from build123d import *

# Parameters (mm, degrees)
F0_R     = 76.2
F1_DEPTH = 25.4
F3_DEPTH = 25.4


with BuildPart() as f1:
    # F0 (on Front) → F1 (new body)
    with BuildSketch(Plane.XZ):
        Circle(F0_R)
    extrude(amount=F1_DEPTH)

    # F2 (on face) → F3 (cut)
    with BuildSketch(Plane.XZ.offset(25.4)):
        with BuildLine():
            Line((-52.494522, 25.127975), (-38.677355, 18.514))
            ThreePointArc((-38.677355, 18.514), (-35.080153, 18.213926), (-32.19177, 20.37891))
            ThreePointArc((-32.19177, 20.37891), (-26.940768, 26.940768), (-20.37891, 32.19177))
            ThreePointArc((-20.37891, 32.19177), (-18.213926, 35.080153), (-18.514, 38.677355))
            Line((-18.514, 38.677355), (-25.127975, 52.494522))
            ThreePointArc((-25.127975, 52.494522), (-28.231073, 55.161107), (-32.293557, 54.675188))
            ThreePointArc((-32.293557, 54.675188), (-44.901281, 44.901281), (-54.675188, 32.293557))
            ThreePointArc((-54.675188, 32.293557), (-55.161107, 28.231073), (-52.494522, 25.127975))
        make_face()
        with BuildLine():
            Line((19.351072, -54.887394), (14.257645, -40.440395))
            ThreePointArc((14.257645, -40.440395), (11.926223, -37.684605), (8.352953, -37.173084))
            ThreePointArc((8.352953, -37.173084), (0, -38.1), (-8.352953, -37.173084))
            ThreePointArc((-8.352953, -37.173084), (-11.926223, -37.684605), (-14.257645, -40.440395))
            Line((-14.257645, -40.440395), (-19.351072, -54.887394))
            ThreePointArc((-19.351072, -54.887394), (-19.04241, -58.967176), (-15.826203, -61.496189))
            ThreePointArc((-15.826203, -61.496189), (0, -63.5), (15.826203, -61.496189))
            ThreePointArc((15.826203, -61.496189), (19.04241, -58.967176), (19.351072, -54.887394))
        make_face()
        with BuildLine():
            Line((25.127975, 52.494522), (18.514, 38.677355))
            ThreePointArc((18.514, 38.677355), (18.213926, 35.080153), (20.37891, 32.19177))
            ThreePointArc((20.37891, 32.19177), (26.940768, 26.940768), (32.19177, 20.37891))
            ThreePointArc((32.19177, 20.37891), (35.080153, 18.213926), (38.677355, 18.514))
            Line((38.677355, 18.514), (52.494522, 25.127975))
            ThreePointArc((52.494522, 25.127975), (55.161107, 28.231073), (54.675188, 32.293557))
            ThreePointArc((54.675188, 32.293557), (44.901281, 44.901281), (32.293557, 54.675188))
            ThreePointArc((32.293557, 54.675188), (28.231073, 55.161107), (25.127975, 52.494522))
        make_face()
    extrude(amount=-F3_DEPTH, mode=Mode.SUBTRACT)


solid = f1.part
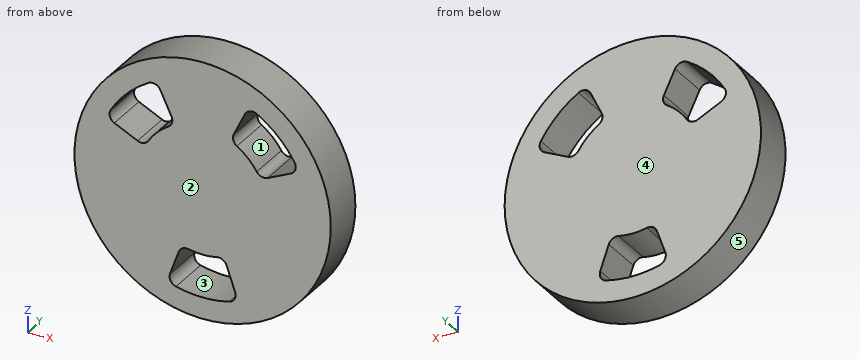
Could you check a few things on this model? Use its own coordinates, in mm. Face numbers are marked on the shaded views. A direction names the side the tool comes from. Give positions to 0.01 mm unless a question says otherwise; leave off trailing zeros. Order: outer loops, then holes, each group sorted by start corner. A loop starts at its lowest first (then second) coordinate and runs counter-clockwise, first axis right, second up.
1. I need wall thicknesses on L1, parallel to X at y = -20.25, z = 41; L2, parallel to X at y = -11.75, z = 30.5; L3, parallel to Z at x = 33, y = -1.75. Which ranges of each line are inside material? Lowest first, please.
Answers below:
L1: x = -64.23 to -48.49, -19.63 to 19.63, 48.49 to 64.23
L2: x = -69.83 to -55.32, -22.83 to 22.83, 55.32 to 69.83
L3: z = -68.68 to 19.4, 54.25 to 68.68
2. Suppose I cut it at A-A (x = 0). Write out the boundary of the cut face in (y, z), plus the area to 3 significant figures.
Answers below:
outline: (-25.4, -76.2) - (0, -76.2) - (0, -63.5) - (-25.4, -63.5) - close; (-25.4, -38.1) - (0, -38.1) - (0, 76.2) - (-25.4, 76.2) - close
area: 3,230 mm2
3. For pin 1 (1.5 mm diameter, centred on x = -28, y = -21.5, fed in from -Z); pin 2 (1.5 mm diameter, centred on y = -15, z = -47.5, fed in from -X); pin 3 (6 mm diameter, centred on x = 0, y = -12, fed in from +Z), each with a flat end and sliding along its axis, tell me the tip position at first contact or that it passes through.
Answers below:
pin 1: stops at z = -71.16
pin 2: stops at x = -60.17
pin 3: stops at z = 76.2
4. Thinking about a two-plate mould opening in Z: for the marked faces 3, 4 and 5, which applies, +Z half, -Z half, draft (parallel to the pull), parting line (faces both ways), or undercut?
Answers below:
face 3: undercut
face 4: draft
face 5: parting line
5. Suppose I cut it at C-C (x = -44.5). Write out the boundary of the cut face in (y, z).
Answers below:
outline: (-25.4, -61.86) - (0, -61.86) - (0, 21.3) - (-25.4, 21.3) - close; (-25.4, 45.3) - (0, 45.3) - (0, 61.86) - (-25.4, 61.86) - close
6. Suppose I cut it at B-B (y = -5.5). Write out the boundary of the cut face in (x, z), plus the area to 3 significant figures.
Answers below:
outline: circle Ø152.4 at (0, 0); hole (-54.68, 32.29) arc R5.08 ccw to (-52.49, 25.13) - (-38.68, 18.51) arc R5.08 ccw to (-32.19, 20.38) arc R38.1 cw to (-20.38, 32.19) arc R5.08 ccw to (-18.51, 38.68) - (-25.13, 52.49) arc R5.08 ccw to (-32.29, 54.68) arc R63.5 ccw to start; hole (-19.35, -54.89) arc R5.08 ccw to (-15.83, -61.5) arc R63.5 ccw to (15.83, -61.5) arc R5.08 ccw to (19.35, -54.89) - (14.26, -40.44) arc R5.08 ccw to (8.35, -37.17) arc R38.1 cw to (-8.35, -37.17) arc R5.08 ccw to (-14.26, -40.44) - close; hole (18.51, 38.68) arc R5.08 ccw to (20.38, 32.19) arc R38.1 cw to (32.19, 20.38) arc R5.08 ccw to (38.68, 18.51) - (52.49, 25.13) arc R5.08 ccw to (54.68, 32.29) arc R63.5 ccw to (32.29, 54.68) arc R5.08 ccw to (25.13, 52.49) - close
area: 15,700 mm2
7. Which directions (+Z, -Z, +X, -X, +Y, -Y) give clear straight access to the entire face, cutting with the end or side of a thin tool? Please do the marked faces 1 and 2.
Answers below:
face 1: +Y, -Y
face 2: +Z, -Z, +X, -X, -Y
8. Suppose I cut it at D-D (z = -26). Write out the boundary of the cut face in (x, y).
Answers below:
outline: (-71.63, -25.4) - (71.63, -25.4) - (71.63, 0) - (-71.63, 0) - close
